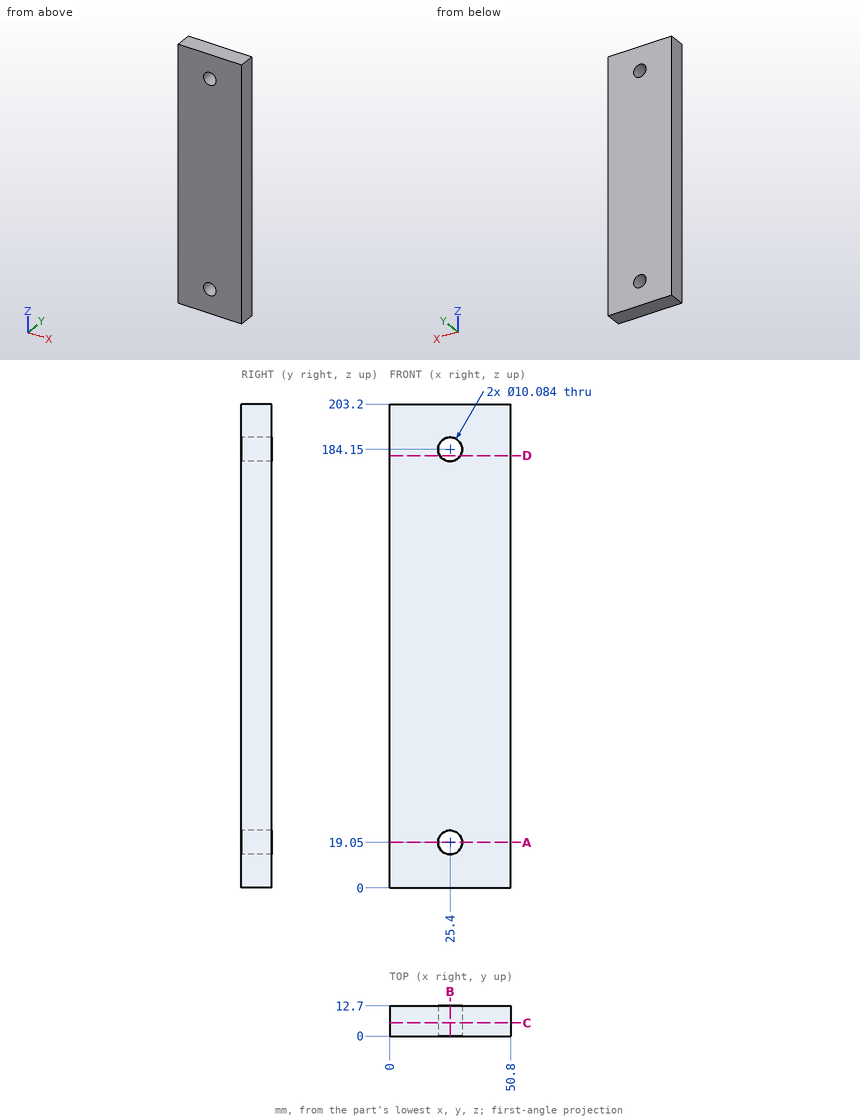
Can you work these out from the drawing? Everything is in mm from the part's minimum corner. Give positions to 0.01 mm unless a question says otherwise; leave off trailing zeros. Loops run counter-clockwise (first coordinate to the right, second up) from the corner with the lowest first, then second, coordinate; pieces in that order, holes last. Notation, with made-up numbers: (35.25, 62) -> (43.25, 62) arc R18 ccw to (43.25, 81) -> close; hole circle Ø10 at (53.25, 51). An arc over 180 degrees is marked (long way). Return JSON: item names as keys, results as strings.
Item 1: If we section it at C-C on y = 5.5: List the corners of the cut face in (x, z) for me, plus the area to 3 significant figures.
Geometry results:
{"outline": "(0, 0) -> (50.8, 0) -> (50.8, 203.2) -> (0, 203.2) -> close; hole circle Ø10.08 at (25.4, 19.05); hole circle Ø10.08 at (25.4, 184.15)", "area": "10,200 mm²"}
Item 2: I need wall thicknesses on L1, parallel to Z at x = 25.4, y = 7.75; L2, parallel to X at y = 9.75, z = 184.15; L3, parallel to Z at x = 24, y = 6. Which ranges of each line are inside material? Lowest first, please. Write a range as from..to.
Geometry results:
{"L1": "z = 0..14.01, 24.09..179.11, 189.19..203.2", "L2": "x = 0..20.36, 30.44..50.8", "L3": "z = 0..14.21, 23.89..179.31, 188.99..203.2"}
Item 3: If we section it at D-D on z = 181.5: List the corners of the cut face in (x, y) for me.
Geometry results:
{"outline": "(0, 0) -> (21.11, 0) -> (21.11, 12.7) -> (0, 12.7) -> close; (29.69, 0) -> (50.8, 0) -> (50.8, 12.7) -> (29.69, 12.7) -> close"}
Item 4: If we section it at B-B on x = 25.4: List the corners of the cut face in (y, z) for me, plus the area to 3 significant figures.
Geometry results:
{"outline": "(0, 0) -> (12.7, 0) -> (12.7, 14.01) -> (0, 14.01) -> close; (0, 24.09) -> (12.7, 24.09) -> (12.7, 179.11) -> (0, 179.11) -> close; (0, 189.19) -> (12.7, 189.19) -> (12.7, 203.2) -> (0, 203.2) -> close", "area": "2,320 mm²"}
Item 5: If we section it at A-A on z = 19.05: List the corners of the cut face in (x, y) for me.
Geometry results:
{"outline": "(0, 0) -> (20.36, 0) -> (20.36, 12.7) -> (0, 12.7) -> close; (30.44, 0) -> (50.8, 0) -> (50.8, 12.7) -> (30.44, 12.7) -> close"}
